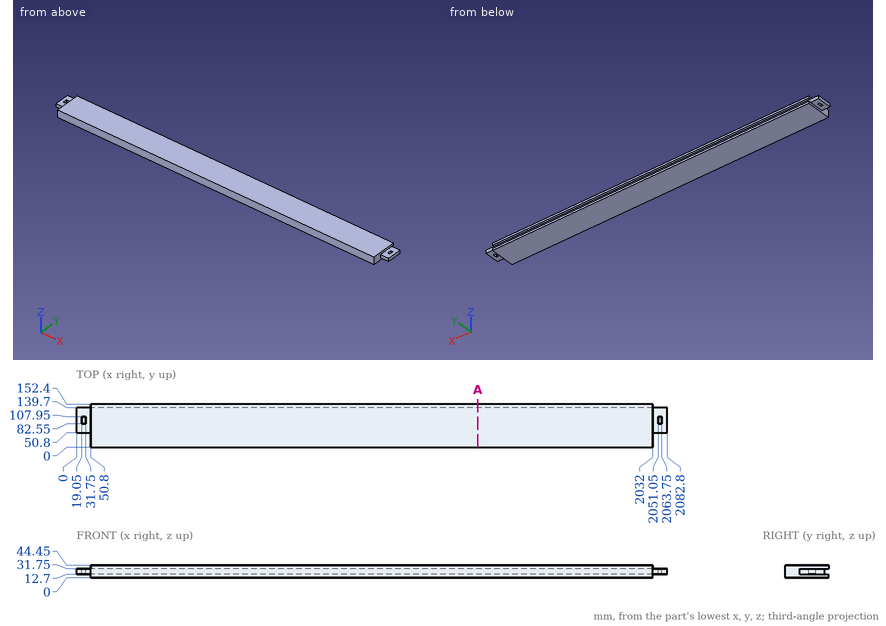
For this review, use the dimensioned drawing (mm, ordinates from the lowest corner) and the shaded views. Round coordinates to 2 decimals unless told otherwise and drop trailing zeros. Write each loop counter-clockwise with the first axis right and the second up, starting at its lowest first coordinate (ties: lowest second). Pieces come first, ordered by that corner, then holes. Notation, with made-up numbers: (17, 26) - (75, 26) arc R19 ccw to (75, 42) - close; hole circle Ø9 at (-7, -27.75). An arc over 180 degrees is marked (long way). One line per item, written item: value. Start each with the question number.
1. Clearance check with flat-ended pins moving along their axes: P1, Ø5.5, axis at x = 32.5, z = 22.5, coming from the -Y side; P2, Ø9.5, axis at x = 1065.5, z = 24, coming from the +Y side; P3, Ø3, axis at x = 1389.5, y = 98, coming from the -Z side; P4, Ø15, axis at x = 23, y = 109.5, coming from the -Z side. State where each tip first meets the part, or that it passes through.
2. Consider section A-A on x = 1415.5. Write out the cut boundary in (y, z).
3. To check wall thickness, follow L1, parallel to X at y = 90.5, z = 19; L2, parallel to X at y = 90, z = 35; L3, parallel to Y at x = 192, z = 14. State the ranges of each line that lie inside material, in increasing order. Write a range as from..to.
Checks:
1. P1: stops at y = 50.8
1. P2: stops at y = 139.7
1. P3: stops at z = 0
1. P4: stops at z = 12.7
2. outline: (0, 0) - (152.4, 0) - (152.4, 12.7) - (139.7, 12.7) - (139.7, 31.75) - (152.4, 31.75) - (152.4, 44.45) - (0, 44.45) - close
3. L1: x = 0..19.05, 31.75..2051.05, 2063.75..2082.8
3. L2: x = 50.8..2032
3. L3: y = 0..139.7
